from build123d import *

# Parameters (mm, degrees)
SKETCH1_R           = 11.938
SKETCH1_R_2         = 8.763
BOSS_EXTRUDE1_DEPTH = 5.08
SKETCH2_R           = 11.938
BOSS_EXTRUDE2_DEPTH = 2.54
BOSS_EXTRUDE8_DEPTH = 2.54


with BuildPart() as part:
    # Sketch1 → Boss-Extrude1 (new body)
    with BuildSketch(Plane.XY):
        Circle(SKETCH1_R)
        Circle(SKETCH1_R_2, mode=Mode.SUBTRACT)
    extrude(amount=BOSS_EXTRUDE1_DEPTH)

    # Sketch2 → Boss-Extrude2 (add)
    with BuildSketch(Plane.XY.offset(5.08)):
        Circle(SKETCH2_R)
    extrude(amount=BOSS_EXTRUDE2_DEPTH)

    # Sketch3 → Boss-Extrude8 (add)
    with BuildSketch(Plane.XY.offset(7.62)):
        with BuildLine():
            Line((1.384866851, 7.764949028), (-1.384866851, 7.764949028))
            Line((-1.384866851, 7.764949028), (-1.384866851, 6.420894347))
            Line((-1.384866851, 6.420894347), (-2.702727896, 6.420894347))
            Line((-2.702727896, 6.420894347), (-2.702727896, 7.764949028))
            Line((-2.702727896, 7.764949028), (-3.54067733, 7.764949028))
            ThreePointArc((-3.54067733, 7.764949028), (-3.845533247, 7.616635469), (-4.019746325, 7.325802449))
            Line((-4.019746325, 7.325802449), (-4.019746325, 4.185239036))
            ThreePointArc((-4.019746325, 4.185239036), (-3.580344494, 3.383503573), (-2.702727896, 3.127295005))
            Line((-2.702727896, 3.127295005), (-2.702727896, -0.115652291))
            ThreePointArc((-2.702727896, -0.115652291), (-3.121575281, -1.926106842), (-4.019746325, -3.552903568))
            Line((-4.019746325, -3.552903568), (-4.019746325, -4.820747752))
            Line((-4.019746325, -4.820747752), (-5.357231947, -4.820747752))
            Line((-5.357231947, -4.820747752), (-5.357231947, -7.568020311))
            Line((-5.357231947, -7.568020311), (5.293156983, -7.568020311))
            Line((5.293156983, -7.568020311), (5.293156983, -4.820747752))
            Line((5.293156983, -4.820747752), (4.019746325, -4.820747752))
            Line((4.019746325, -4.820747752), (4.019746325, -3.552903568))
            ThreePointArc((4.019746325, -3.552903568), (3.121575281, -1.926106842), (2.702727896, -0.115652291))
            Line((2.702727896, -0.115652291), (2.702727896, 3.127295005))
            ThreePointArc((2.702727896, 3.127295005), (3.580344494, 3.383503573), (4.019746325, 4.185239036))
            Line((4.019746325, 4.185239036), (4.019746325, 7.325802449))
            ThreePointArc((4.019746325, 7.325802449), (3.845533247, 7.616635469), (3.54067733, 7.764949028))
            Line((3.54067733, 7.764949028), (2.702727896, 7.764949028))
            Line((2.702727896, 7.764949028), (2.702727896, 6.420894347))
            Line((2.702727896, 6.420894347), (1.384866851, 6.420894347))
            Line((1.384866851, 6.420894347), (1.384866851, 7.764949028))
        make_face()
    extrude(amount=BOSS_EXTRUDE8_DEPTH)


solid = part.part
Input: part model. Units: mm. Frame: model coordinates. A direction names the side the tool comes from. Round coordinates to 2 decimals unless told otherwise and drop trailing zeros. Write each loop counter-clockwise with the first axis right and the second up, starting at its lowest first coordinate (ties: lowest second). Pieces come first, ordered by that corner, then holes.
1) Cut plane D-D (z = 3.25). Return the cut outline in (x, y), then the cut area to 3 significant figures.
2) Ray query, L1, parallel to Y at x = 0, z = 1.6; L2, parallel to Z at x = -3, y = 1; L3, parallel to Y at x = -4.75, z = 3. Return the intervals inside material, ascending.
3) Contact query for flat-ended pins moving along their axis: P1, Ø1.5, axis at y = 7, z = 9.5, coming from the +X side; P2, Ø0.7, axis at y = 7, z = 9.5, coming from the -X side; P3, Ø3, axis at y = 5, z = 5.5, coming from the -X side; P4, Ø10, axis at x = -4.5, y = -3, coming from the +Z side. Output: stop coordinate, or through.
4) Cut plane B-B (x = 0). Return the cut outline in (y, z).
5) Cut plane A-A (z = 8.5). Return the cut outline in (x, y), then the cut area to 3 significant figures.
6) Cut plane C-C (y = -2.25). Return the cut outline in (x, z).
7) Draft query along X for faces 4 (the flat face through (-2, 6.421, 9)), 5 (the flat face through (-4, 8, 0)), 6 (the flat face through (2.703, 1, 9)), 7 (the cylindrical face through (8.36, 2.63, 2.5)). Return one class per face: pulls with the +X half, pulls with the -X half, needs draft (parallel to the pull), parting line crosses it, or undercut.
8) Reachability of faces 1 (the flat face through (4.02, 6, 9)), 2 (the flat face through (-2.703, 7, 9)), 3 (the flat face through (-3, 7.765, 9)) from +Z, -Z, +X, -X, +Y, -Y: full face, straight path, thin tool, end or side. Return the list, or none.
Geometry says:
1. outline: circle Ø23.88 at (0, 0); hole circle Ø17.53 at (0, 0)
1. area: 206 mm2
2. L1: y = -11.94 to -8.76, 8.76 to 11.94
2. L2: z = 5.08 to 7.62
2. L3: y = -10.95 to -7.36, 7.36 to 10.95
3. P1: stops at x = 4.02
3. P2: stops at x = -4.02
3. P3: stops at x = -11.41
3. P4: stops at z = 10.16
4. outline: (-11.94, 0) - (-8.76, 0) - (-8.76, 5.08) - (8.76, 5.08) - (8.76, 0) - (11.94, 0) - (11.94, 7.62) - (7.76, 7.62) - (7.76, 10.16) - (-7.57, 10.16) - (-7.57, 7.62) - (-11.94, 7.62) - close
5. outline: (-5.36, -7.57) - (5.29, -7.57) - (5.29, -4.82) - (4.02, -4.82) - (4.02, -3.55) arc R6.73 cw to (2.7, -0.12) - (2.7, 3.13) arc R1.19 ccw to (4.02, 4.19) - (4.02, 7.33) arc R0.59 ccw to (3.54, 7.76) - (2.7, 7.76) - (2.7, 6.42) - (1.38, 6.42) - (1.38, 7.76) - (-1.38, 7.76) - (-1.38, 6.42) - (-2.7, 6.42) - (-2.7, 7.76) - (-3.54, 7.76) arc R0.59 ccw to (-4.02, 7.33) - (-4.02, 4.19) arc R1.19 ccw to (-2.7, 3.13) - (-2.7, -0.12) arc R6.73 cw to (-4.02, -3.55) - (-4.02, -4.82) - (-5.36, -4.82) - close
5. area: 112 mm2
6. outline: (-11.72, 0) - (-8.47, 0) - (-8.47, 5.08) - (8.47, 5.08) - (8.47, 0) - (11.72, 0) - (11.72, 7.62) - (3.26, 7.62) - (3.26, 10.16) - (-3.26, 10.16) - (-3.26, 7.62) - (-11.72, 7.62) - close
7. face 4: undercut
7. face 5: needs draft
7. face 6: pulls with the +X half
7. face 7: undercut
8. face 1: +Z, +X, +Y
8. face 2: +Z, +Y
8. face 3: +Z, +X, -X, +Y
